Could you check a few things on this model? Use its own coordinates, in mm. A direction names the side the tool comes from. Give positions to 0.01 mm unless a question says otherwise; leave off trailing zeros. Order: outer loops, then holes, each group sorted by start corner. A loop starts at its lowest first (then second) coordinate and runs counter-clockwise, first axis right, second up. Notation, with made-up numbers: (77, 36.5) -> (115, 36.5) arc R11 ccw to (115, 46.5) -> close; hole circle Ø4 at (31, 23). An arc over 180 degrees is marked (long way). One line per item, written item: value.
```python
from build123d import *

# Parameters (mm, degrees)
F0_R     = 6.5
F1_DEPTH = 5
F3_DEPTH = 10


with BuildPart() as f1:
    # F0 (on Front) → F1 (new body, symmetric)
    with BuildSketch(Plane.XZ):
        with BuildLine():
            Line((-12.679406, 22.584124), (-10.90092, 18.589579))
            ThreePointArc((-10.90092, 18.589579), (-12.666772, 17.434316), (-14.311171, 16.111887))
            Line((-14.311171, 16.111887), (-17.560627, 19.03771))
            ThreePointArc((-17.560627, 19.03771), (-21.030999, 18.936396), (-20.769004, 15.474445))
            Line((-20.769004, 15.474445), (-17.519549, 12.548622))
            ThreePointArc((-17.519549, 12.548622), (-18.662847, 10.775), (-19.6272, 8.898063))
            Line((-19.6272, 8.898063), (-23.785765, 10.249263))
            ThreePointArc((-23.785765, 10.249263), (-26.914899, 8.745181), (-25.267454, 5.689094))
            Line((-25.267454, 5.689094), (-21.108888, 4.337894))
            ThreePointArc((-21.108888, 4.337894), (-21.431947, 2.252588), (-21.549508, 0.145684))
            Line((-21.549508, 0.145684), (-25.898128, -0.311375))
            ThreePointArc((-25.898128, -0.311375), (-28.14497, -2.958156), (-25.39693, -5.079953))
            Line((-25.39693, -5.079953), (-21.04831, -4.622895))
            ThreePointArc((-21.04831, -4.622895), (-20.495268, -6.659316), (-19.74571, -8.631886))
            Line((-19.74571, -8.631886), (-23.53247, -10.818173))
            ThreePointArc((-23.53247, -10.818173), (-24.508519, -14.15), (-21.135047, -14.97063))
            Line((-21.135047, -14.97063), (-17.348287, -12.784343))
            ThreePointArc((-17.348287, -12.784343), (-16.014771, -14.419765), (-14.527699, -15.916924))
            Line((-14.527699, -15.916924), (-17.097834, -19.45441))
            ThreePointArc((-17.097834, -19.45441), (-16.634323, -22.895181), (-13.218722, -22.27275))
            Line((-13.218722, -22.27275), (-10.648588, -18.735263))
            ThreePointArc((-10.648588, -18.735263), (-8.765175, -19.686905), (-6.797718, -20.449781))
            Line((-6.797718, -20.449781), (-7.706827, -24.726804))
            ThreePointArc((-7.706827, -24.726804), (-5.883901, -27.681577), (-3.01676, -25.723708))
            Line((-3.01676, -25.723708), (-2.107651, -21.446685))
            ThreePointArc((-2.107651, -21.446685), (0, -21.55), (2.107651, -21.446685))
            Line((2.107651, -21.446685), (3.01676, -25.723708))
            ThreePointArc((3.01676, -25.723708), (5.883901, -27.681577), (7.706827, -24.726804))
            Line((7.706827, -24.726804), (6.797718, -20.449781))
            ThreePointArc((6.797718, -20.449781), (8.765175, -19.686905), (10.648588, -18.735263))
            Line((10.648588, -18.735263), (13.218722, -22.27275))
            ThreePointArc((13.218722, -22.27275), (16.634323, -22.895181), (17.097834, -19.45441))
            Line((17.097834, -19.45441), (14.527699, -15.916924))
            ThreePointArc((14.527699, -15.916924), (16.014771, -14.419765), (17.348287, -12.784343))
            Line((17.348287, -12.784343), (21.135047, -14.97063))
            ThreePointArc((21.135047, -14.97063), (24.508519, -14.15), (23.53247, -10.818173))
            Line((23.53247, -10.818173), (19.74571, -8.631886))
            ThreePointArc((19.74571, -8.631886), (20.495268, -6.659316), (21.04831, -4.622895))
            Line((21.04831, -4.622895), (25.39693, -5.079953))
            ThreePointArc((25.39693, -5.079953), (28.14497, -2.958156), (25.898128, -0.311375))
            Line((25.898128, -0.311375), (21.549508, 0.145684))
            ThreePointArc((21.549508, 0.145684), (21.431947, 2.252588), (21.108888, 4.337894))
            Line((21.108888, 4.337894), (25.267454, 5.689094))
            ThreePointArc((25.267454, 5.689094), (26.914899, 8.745181), (23.785765, 10.249263))
            Line((23.785765, 10.249263), (19.6272, 8.898063))
            ThreePointArc((19.6272, 8.898063), (18.662847, 10.775), (17.519549, 12.548622))
            Line((17.519549, 12.548622), (20.769004, 15.474445))
            ThreePointArc((20.769004, 15.474445), (21.030999, 18.936396), (17.560627, 19.03771))
            Line((17.560627, 19.03771), (14.311171, 16.111887))
            ThreePointArc((14.311171, 16.111887), (12.666772, 17.434316), (10.90092, 18.589579))
            Line((10.90092, 18.589579), (12.679406, 22.584124))
            ThreePointArc((12.679406, 22.584124), (11.510647, 25.853336), (8.299097, 24.534364))
            Line((8.299097, 24.534364), (6.520611, 20.539818))
            ThreePointArc((6.520611, 20.539818), (4.480497, 21.079081), (2.397423, 21.416229))
            Line((2.397423, 21.416229), (2.397423, 25.788803))
            ThreePointArc((2.397423, 25.788803), (0, 28.3), (-2.397423, 25.788803))
            Line((-2.397423, 25.788803), (-2.397423, 21.416229))
            ThreePointArc((-2.397423, 21.416229), (-4.480497, 21.079081), (-6.520611, 20.539818))
            Line((-6.520611, 20.539818), (-8.299097, 24.534364))
            ThreePointArc((-8.299097, 24.534364), (-11.510647, 25.853336), (-12.679406, 22.584124))
        make_face()
        Circle(F0_R, mode=Mode.SUBTRACT)
    extrude(amount=F1_DEPTH, both=True)

    # F2 (on face) → F3 (cut)
    with BuildSketch(Plane.XZ.offset(5)):
        with BuildLine():
            ThreePointArc((-5.755287, 18.159823), (-13.470384, 13.470384), (-18.159823, 5.755287))
            ThreePointArc((-18.159823, 5.755287), (-17.793847, 3.523216), (-15.776644, 2.5))
            Line((-15.776644, 2.5), (-9.54669, 2.5))
            ThreePointArc((-9.54669, 2.5), (-8.252423, 2.861104), (-7.332049, 3.8401))
            ThreePointArc((-7.332049, 3.8401), (-5.852577, 5.852577), (-3.8401, 7.332049))
            ThreePointArc((-3.8401, 7.332049), (-2.861104, 8.252423), (-2.5, 9.54669))
            Line((-2.5, 9.54669), (-2.5, 15.776644))
            ThreePointArc((-2.5, 15.776644), (-3.523216, 17.793847), (-5.755287, 18.159823))
        make_face()
        with BuildLine():
            ThreePointArc((5.755287, 18.159823), (3.523216, 17.793847), (2.5, 15.776644))
            Line((2.5, 15.776644), (2.5, 9.54669))
            ThreePointArc((2.5, 9.54669), (2.861104, 8.252423), (3.8401, 7.332049))
            ThreePointArc((3.8401, 7.332049), (5.852577, 5.852577), (7.332049, 3.8401))
            ThreePointArc((7.332049, 3.8401), (8.252423, 2.861104), (9.54669, 2.5))
            Line((9.54669, 2.5), (15.776644, 2.5))
            ThreePointArc((15.776644, 2.5), (17.793847, 3.523216), (18.159823, 5.755287))
            ThreePointArc((18.159823, 5.755287), (13.470384, 13.470384), (5.755287, 18.159823))
        make_face()
        with BuildLine():
            Line((-9.54669, -2.5), (-15.776644, -2.5))
            ThreePointArc((-15.776644, -2.5), (-17.793847, -3.523216), (-18.159823, -5.755287))
            ThreePointArc((-18.159823, -5.755287), (-13.470384, -13.470384), (-5.755287, -18.159823))
            ThreePointArc((-5.755287, -18.159823), (-3.523216, -17.793847), (-2.5, -15.776644))
            Line((-2.5, -15.776644), (-2.5, -9.54669))
            ThreePointArc((-2.5, -9.54669), (-2.861104, -8.252423), (-3.8401, -7.332049))
            ThreePointArc((-3.8401, -7.332049), (-5.852577, -5.852577), (-7.332049, -3.8401))
            ThreePointArc((-7.332049, -3.8401), (-8.252423, -2.861104), (-9.54669, -2.5))
        make_face()
        with BuildLine():
            Line((2.5, -7.890204), (2.5, -15.776644))
            ThreePointArc((2.5, -15.776644), (3.523216, -17.793847), (5.755287, -18.159823))
            ThreePointArc((5.755287, -18.159823), (13.470384, -13.470384), (18.159823, -5.755287))
            ThreePointArc((18.159823, -5.755287), (17.793847, -3.523216), (15.776644, -2.5))
            Line((15.776644, -2.5), (9.54669, -2.5))
            ThreePointArc((9.54669, -2.5), (8.252423, -2.861104), (7.332049, -3.8401))
            ThreePointArc((7.332049, -3.8401), (5.316778, -6.343278), (2.5, -7.890204))
        make_face()
    extrude(amount=-F3_DEPTH, mode=Mode.SUBTRACT)


solid = f1.part
```
1) Suppose I cut it at A-A, the plane x = 0. Write out the boundary of the cut face in (y, z), then the cut area to 4 significant figures.
Answer below:
outline: (-5, -21.55) -> (5, -21.55) -> (5, -6.5) -> (-5, -6.5) -> close; (-5, 6.5) -> (5, 6.5) -> (5, 28.3) -> (-5, 28.3) -> close
area: 368.5 mm2
2) Suppose I cut it at C-C, the plane y = 3.25. State how many separate pieces and enclosed holes the cut face has, then the cut area to 3 significant figures.
Answer below:
separate pieces: 1
enclosed holes: 5
area: 1,090 mm2
3) We'd pull the mould along X, two halves only. Please class faces 4 (the flat face through (23.159, -0.07, 5.004)), 5 (the cylindrical face through (-0.03, -0.07, -21.55)), 6 (the flat face through (-23.69, -0.07, -0.08)): +X half, -X half, draft (parallel to the pull), parting line (faces both ways), or undercut.
Answer below:
face 4: +X half
face 5: undercut
face 6: -X half
4) Suppose I cut it at B-B, the plane z = 1.5. Write out the boundary of the cut face in (x, y).
Answer below:
outline: (-21.5, -5) -> (-6.32, -5) -> (-6.32, 5) -> (-21.5, 5) -> close; (6.32, -5) -> (21.5, -5) -> (21.5, 5) -> (6.32, 5) -> close
5) For faces 1 (the flat face through (11.916, -0.07, -20.479)), 2 (the cylindrical face through (-2.87, -0.07, 8.24)), 3 (the flat face through (15.959, -0.07, 17.595)), which set-ups out of +Z, -Z, +X, -X, +Y, -Y let a thin tool reach every point of the face, with its end or its side?
Answer below:
face 1: -Z, +Y, -Y
face 2: +Y, -Y
face 3: +Z, +Y, -Y
6) For P1, Ø5, axis at x = 14, y = 1, coming from the +Z side; P2, Ø1.9, axis at x = 12.5, y = 1, coming from the -Z side; P3, Ø2, axis at y = -1, z = 22.5, coming from the -X side; P4, Ø11.5, axis at x = 0, z = 0, coming from the +Y side, each with a flat end and sliding along its axis, tell me the tip position at first contact or that it passes through.
Answer below:
P1: stops at z = 25.86
P2: stops at z = -22.57
P3: stops at x = -12.93
P4: passes through
7) If I drill on line 1 along Z through (x, y) = (-12, -0.5); line 2 along X through (y, z) = (-2, 12); line 3 along X through (y, z) = (2.5, 17.5), over which ranges is the centre line in solid material (lowest first)?
Answer below:
line 1: z = -20.6 to -14.8, -2.5 to 2.5, 14.8 to 17.9, 21.06 to 25.56
line 2: x = -17.9 to -14.8, -2.5 to 2.5, 14.8 to 17.9
line 3: x = -21.64 to -15.85, -12.58 to -7.53, -3.19 to 3.19, 7.53 to 12.58, 15.85 to 21.64
